Check sheet for the drawn part. Datum: minimum x, y, z corner. Units: mm. Round coordinates to 2 decimals unless told otherwise and drop trailing zeros. Order: outer loops, then holes, each group sorted by start corner. A loop starts at its lowest first (then second) coordinate and runs counter-clockwise, first axis right, second up. Notation, with made-up numbers: (-20.75, 39.25) -> (-3.75, 39.25) arc R9 ccw to (-3.75, 55.25) -> close; hole circle Ø6 at (85.5, 16.25). An arc over 180 degrees is marked (long way). Answer in a Markdown table with one row per item.
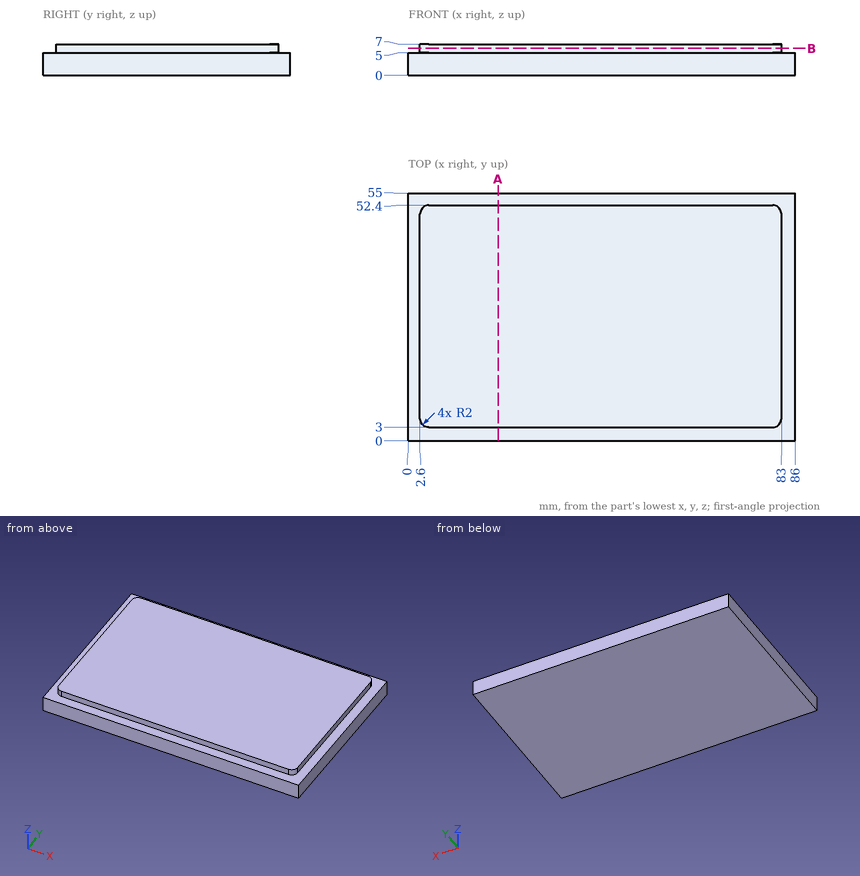
(1) Section check B-B on z = 6. Record the boundary of the cut face in (x, y).
Solutions:
| item | result |
|---|---|
| outline | (2.6, 5) arc R2 ccw to (4.6, 3) -> (81, 3) arc R2 ccw to (83, 5) -> (83, 50.4) arc R2 ccw to (81, 52.4) -> (4.6, 52.4) arc R2 ccw to (2.6, 50.4) -> close |
(2) Section check A-A on x = 20. Record the boundary of the cut face in (y, z), plus the area to 3 significant figures.
Solutions:
| item | result |
|---|---|
| outline | (0, 0) -> (55, 0) -> (55, 5) -> (52.4, 5) -> (52.4, 7) -> (3, 7) -> (3, 5) -> (0, 5) -> close |
| area | 374 mm^2 |
(3) Scan lines: probe 1 along X at (y, z) = (38.5, 6.5); probe 2 along Y at (x, z) = (29, 5.75). Record each from-to range of solid material in increasing order. Write a range as from..to.
Solutions:
| item | result |
|---|---|
| probe 1 | 2.6..83 |
| probe 2 | 3..52.4 |
(4) Depth check by flat-ended pin: pin 1 Ø1.6 at (y, z) = (18, 6) entering from +X; pin 2 Ø0.6 at (x, z) = (43.5, 6) entering from +Y; pin 3 Ø1.6 at (x, z) = (59, 6) entering from -Y. Enter the tip coordinate at first touch or a pass-through.
Solutions:
| item | result |
|---|---|
| pin 1 | x = 83 |
| pin 2 | y = 52.4 |
| pin 3 | y = 3 |
